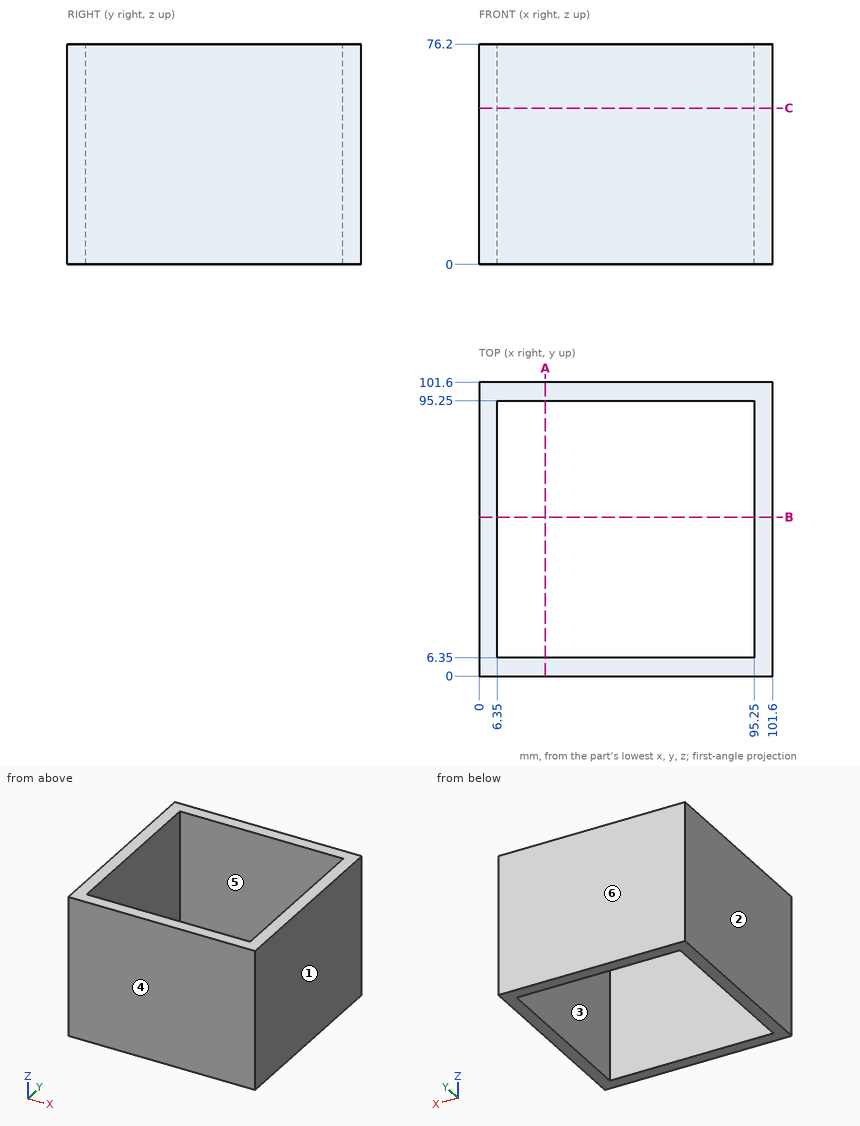
Here's the drawing with two shaded views (mm, measured from the low corner). I have some questions. A direction names the side the tool comes from. Round coordinates to 2 decimals unless told otherwise and drop trailing zeros. Write each loop counter-clockwise with the first axis right and the second up, starting at its lowest first coordinate (ties: lowest second). Pieces come first, ordered by that corner, then holes. Notation, with made-up numbers: M 86.25,63 L 140.25,63 A17 ccw 140.25,77 Z; hole C 22.25,44 d9. An arc over 180 degrees is marked long. Use CSV: the item, a comma, the result in double quotes.
(1) Imagine slicing it at C-C (z = 54). Write out the boundary of the cut face in (x, y).
Check values:
outline,"M 0,0 L 101.6,0 L 101.6,101.6 L 0,101.6 Z; hole M 6.35,6.35 L 95.25,6.35 L 95.25,95.25 L 6.35,95.25 Z"
(2) On a 3-axis mill with a long thin cutter (end or side, diameter ignored), from which of +Z, -Z, +X, -X, +Y, -Y can I reach the whole of each face in a straight line? I mean the marked faces 5 and 6. Say none if no direction works.
Check values:
face 5,"+Z, -Z"
face 6,"+Z, -Z, +X, -X, +Y"
(3) Imagine slicing it at A-A (x = 23). Write out the boundary of the cut face in (y, z), plus the area to 3 significant figures.
Check values:
outline,"M 0,0 L 6.35,0 L 6.35,76.2 L 0,76.2 Z; M 95.25,0 L 101.6,0 L 101.6,76.2 L 95.25,76.2 Z"
area,"968 mm^2"
(4) I need wall thicknesses on line 1 along X through (y, z) = (92, 11). Which ranges of the line are inside material? Lowest first, please.
Check values:
line 1,"0 to 6.35, 95.25 to 101.6"
(5) We'd pull the mould along X, two halves only. Please class the marked faces 1, 2, 3 and 4: +X half, -X half, draft (parallel to the pull), parting line (faces both ways), or undercut.
Check values:
face 1,"+X half"
face 2,"-X half"
face 3,"undercut"
face 4,"draft"
